Check sheet for the modelled part. Datum: model origin and axes. Units: mm. Face numbers are marked on the shaded views. Give positions to 0.01 mm unless a question says otherwise; leave off trailing zeros. Loops run counter-clockwise (first coordinate to the right, second up) from the corner with the lowest first, then second, coordinate; pieces in that order, holes last. Notation, with made-up numbers: M -32,69 L 1,69 A31 ccw 1,104 Z; hole C 11.25,79 d1. An arc over 180 degrees is marked long. Write each question's results on one line, items separated by ' | '. Start each with the question number.
1. Go/stop test with flat-tipped pins: pin 1 (4 mm diameter, centred on x = -1, z = -8, fed in from +Y); pin 2 (4.5 mm diameter, centred on x = 30, y = -40, fed in from +Z). Record where each tip stops, or that it passes through.
2. Sectioned sample at C-C on z = -4. Record the cut outline in (x, y).
3. Draft check along Z on the marked faces 1, 2 and 3. Enter one of: pulls with the +Z half, pulls with the -Z half, needs draft (parallel to the pull), parting line crosses it, or undercut.
4. Sectioned sample at A-A on z = 0. Record the cut outline in (x, y), and give its area (3 significant figures).
5. Sectioned sample at B-B on y = -15.5. Record the cut outline in (x, z), and give its area (3 significant figures).
6. Material ranges on line 1 along X through (y, z) = (-40, 13.5); line 2 along Y through (x, z) = (30, 11); line 3 along X through (y, z) = (-12.5, -5.5), recorded low to high.
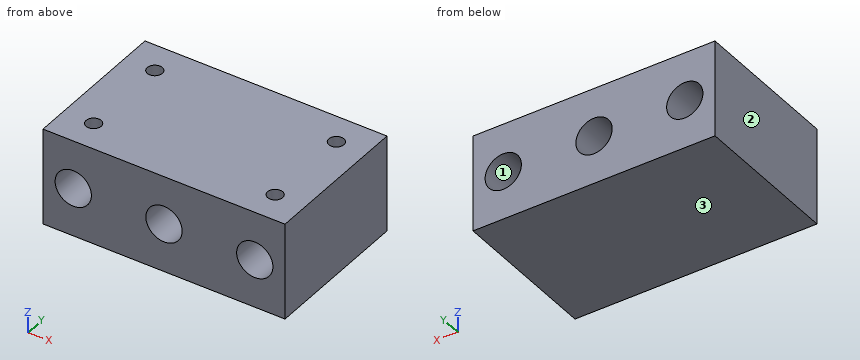
```python
from build123d import *

# Parameters (mm, degrees)
F0_W     = 80
F0_H     = 32
F0_R     = 6
F1_DEPTH = 50
F3_D     = 5
F3_DEPTH = 8
F3_TIP   = 1.5021515476


with BuildPart() as f1:
    # F0 (on Front) → F1 (new body)
    with BuildSketch(Plane.XZ):
        Rectangle(F0_W, F0_H)
        with Locations((-30, 0)):
            Circle(F0_R, mode=Mode.SUBTRACT)
        Circle(F0_R, mode=Mode.SUBTRACT)
        with Locations((30, 0)):
            Circle(F0_R, mode=Mode.SUBTRACT)
    extrude(amount=F1_DEPTH)

    # F3
    with Locations(Plane.XY.offset(16)):
        with Locations((-30, -40), (-30, -10), (30, -40), (30, -10)):
            Hole(F3_D / 2, depth=F3_DEPTH)
            with Locations((0, 0, -(F3_DEPTH + F3_TIP / 2))):  # 118° drill point
                Cone(0, F3_D / 2, F3_TIP, mode=Mode.SUBTRACT)


solid = f1.part
```
Output values:
1) pin 1: y = 0 | pin 2: z = 7.85
2) outline: M -40,-50 L -34.47,-50 L -34.47,0 L -40,0 Z; M -25.53,-50 L -4.47,-50 L -4.47,0 L -25.53,0 Z; M 4.47,-50 L 25.53,-50 L 25.53,0 L 4.47,0 Z; M 34.47,-50 L 40,-50 L 40,0 L 34.47,0 Z
3) face 1: undercut | face 2: needs draft | face 3: pulls with the -Z half
4) outline: M -40,-50 L -36,-50 L -36,0 L -40,0 Z; M -24,-50 L -6,-50 L -6,0 L -24,0 Z; M 6,-50 L 24,-50 L 24,0 L 6,0 Z; M 36,-50 L 40,-50 L 40,0 L 36,0 Z | area: 2,200 mm2
5) outline: M -40,-16 L 40,-16 L 40,16 L -40,16 Z; hole C -30,0 d12; hole C 0,0 d12; hole C 30,0 d12 | area: 2,220 mm2
6) line 1: -40 to -32.5, -27.5 to 27.5, 32.5 to 40 | line 2: -50 to -42.5, -37.5 to -12.5, -7.5 to 0 | line 3: -40 to -32.4, -27.6 to -2.4, 2.4 to 27.6, 32.4 to 40
